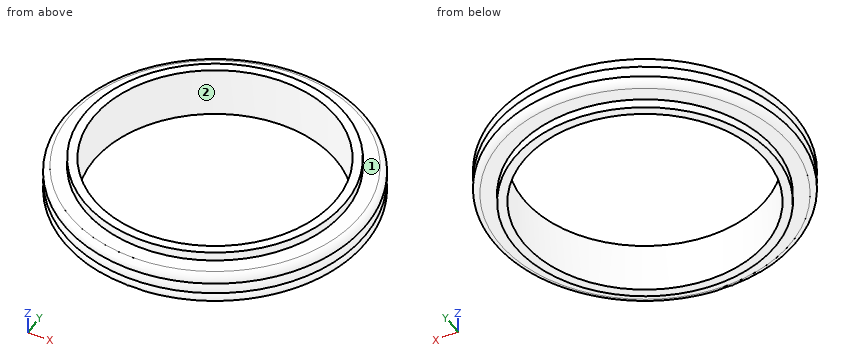
```python
from build123d import *


with BuildPart() as part:
    # Sketch1 → Revolve1 (revolve)
    with BuildSketch(Plane(origin=(0, 0, 0), x_dir=(0, 0, -1), z_dir=(1, 0, 0)), mode=Mode.PRIVATE) as revolve1_sk:
        with BuildLine():
            Line((8.25, 40), (-8.25, 40))
            Line((-8.25, 40), (-8.25, 43))
            Line((-8.25, 43), (-5.25, 43))
            Line((-5.25, 43), (-5.25, 48))
            ThreePointArc((-5.25, 48), (-3.991619849, 49.857417562), (-1.8, 49.377497731))
            ThreePointArc((-1.8, 49.377497731), (0, 49.977497731), (1.8, 49.377497731))
            ThreePointArc((1.8, 49.377497731), (3.991619849, 49.857417562), (5.25, 48))
            Line((5.25, 48), (5.25, 43))
            Line((5.25, 43), (8.25, 43))
            Line((8.25, 43), (8.25, 40))
        make_face()
    revolve(revolve1_sk.sketch.rotate(Axis((0, 0, 0), (0, 0, 1)), 90), axis=Axis((0, 0, 0), (0, 0, 1)))


solid = part.part
```
Can you work these out from the model? Positions are in its coordinate system, mm. Face numbers are marked on the shaded views. Give positions to 0.01 mm unless a question says otherwise; leave off trailing zeros. Order: outer loops, then holes, each group sorted by start corner. A loop starts at its lowest first (then second) coordinate and runs counter-clockwise, first axis right, second up. Notation, with made-up numbers: M 38,85 L 88,85 A18 ccw 88,114 Z; hole C -10,86.5 d7. An arc over 180 degrees is marked long. One line per item, written item: value.
1) For P1, Ø1.5, axis at x = -25.5, z = -4, coming from the +Y side; P2, Ø2, axis at y = 30, z = 2, coming from the -X side; P3, Ø8, axis at x = -1.5, z = -4.5, coming from the -Y side, each with a flat end and sliding along its axis, tell me the tip position at first contact or that it passes through.
Answer sheet:
P1: stops at y = 43.35
P2: stops at x = -40.46
P3: stops at y = -50
2) I want a section at A-A, the plane x = 0. List the corners of the cut face in (y, z) for me.
Answer sheet:
outline: M -49.38,-1.8 A2 ccw -48,-5.25 L -43,-5.25 L -43,-8.25 L -40,-8.25 L -40,8.25 L -43,8.25 L -43,5.25 L -48,5.25 A2 ccw -49.38,1.8 A3 ccw Z; M 40,-8.25 L 43,-8.25 L 43,-5.25 L 48,-5.25 A2 ccw 49.38,-1.8 A3 ccw 49.38,1.8 A2 ccw 48,5.25 L 43,5.25 L 43,8.25 L 40,8.25 Z
3) We'd pull the mould along Y, two halves only. Please class the marked faces 1 and 2: released by +Y, released by -Y, zero draft, split by the parting line, or undercut.
Answer sheet:
face 1: zero draft
face 2: undercut
4) I want a section at C-C, the plane z = 6.5. List the corners of the cut face in (x, y) for me.
Answer sheet:
outline: C 0,0 d86; hole C 0,0 d80
5) Please list where these lines run through material, in increasing order: line 1 along Z through (x, y) = (-34, 36); line 2 along Y through (x, z) = (0, 0.25); line 3 along Y through (x, z) = (-14.5, -6.5).
Answer sheet:
line 1: z = -4.55 to -1.95, -1.6 to 1.6, 1.95 to 4.55
line 2: y = -49.97 to -40, 40 to 49.97
line 3: y = -40.48 to -37.28, 37.28 to 40.48
